Check sheet for the modelled part. Datum: model origin and axes. Units: mm. Face numbers are marked on the shaded views. A direction names the side the tool comes from. Give positions to 0.01 mm unless a question says otherwise; leave off trailing zeros. Write each loop counter-clockwise with the first axis right and the second up, starting at its lowest first coordinate (ties: lowest second). Pieces come first, ordered by that corner, then holes. Notation, with made-up numbers: (15.5, -13) -> (21.5, -13) arc R13 cw to (21.5, 5) -> close; hole circle Ø2 at (34.5, 1). An arc over 180 degrees is marked (long way). Use a Markdown table: item, result. Add a question column.
1. Cross-section at A-A (z = -0.85). Enter the section's corners in (x, y), then the cut area to 3 significant figures.
2. Scan lines: probe 1 along X at (y, z) = (39.5, 1); probe 2 along Y at (x, z) = (129.5, 1.25); probe 3 along X at (y, z) = (46, -0.25). Record each from-to range of solid material in increasing order. Write a range as [from, to].
3. Cross-section at D-D (y = 60.5). Enter the section's corners in (x, z).
4. Cross-section at B-B (x = 31.5). Enter the section's corners in (y, z).
5. Gauge pin test, flat ends, axial feed: P1, Ø1, axis at y = 38.5, z = -1, coming from the -X side; P2, Ø1.2, axis at y = 74, z = 0, coming from the +X side; P3, Ø3.5, axis at x = 3.5, y = 22, coming from the -Z side; P4, Ø1, axis at x = 32, y = 37, coming from the +Z side. Record the tip position at first contact, or that the pin passes through.
6. Set-up check for the marked faces 1 and 2: record each of +Z, -Z, +X, -X, +Y, -Y from which the full face is reachable in a straight line by a thin tool's end or side.
7. Cross-section at C-C (y = 39.5). Enter the section's corners in (x, z), then the cut area to 3 significant figures.
Autodesk Inventor part; units mm, degrees
ref_plane "YZ Plane" through (0, 0, 0) normal (1, 0, 0) x (0, 1, 0)
ref_plane "XZ Plane" through (0, 0, 0) normal (0, 1, 0) x (-1, 0, 0)
ref_plane "XY Plane" through (0, 0, 0) normal (0, 0, 1) x (1, 0, 0)
sketch "Sketch1" plane through (0, 0, 0) normal (0, 0, 1) x (1, 0, 0)
  line L0 (0, 0) -> (123, 0)
  line L1 (123, 0) -> (123, 79)
  line L2 (123, 79) -> (0, 79)
  line L3 (0, 79) -> (0, 0)
  line L4 (12, 79) -> (12, 0)
  line L5 (123, 69.5) -> (126.5, 69.5)
  line L6 (126.5, 69.5) -> (126.5, 9.5)
  line L7 (126.5, 9.5) -> (123, 9.5)
  line L8 (123, 9.5) -> (123, 69.5)
  line L9 (126.5, 9.5) -> (132.5, 9.5)
  line L10 (132.5, 9.5) -> (132.5, 69.5)
  line L11 (132.5, 69.5) -> (126.5, 69.5)
  line L12 (126.5, 69.5) -> (126.5, 9.5)
  line L13 (123, 69.5) -> (119, 69.5)
  line L14 (119, 69.5) -> (119, 79)
  line L15 (119, 79) -> (123, 79)
  line L16 (123, 79) -> (123, 69.5)
  line L17 (123, 9.5) -> (119, 9.5)
  line L18 (119, 9.5) -> (119, 0)
  line L19 (119, 0) -> (123, 0)
  line L20 (123, 0) -> (123, 9.5)
  circle A0 centre (129.5, 39.5) radius 2.1
  line L21 (9, 39.5) -> (5, 39.5) construction
  line L22 (9, 42) -> (5, 42)
  line L23 (5, 37) -> (9, 37)
  arc A1 (9, 37) -> (9, 42) centre (9, 39.5) ccw
  arc A2 (5, 42) -> (5, 37) centre (5, 39.5) ccw
  point P0 (7, 39.5)
  dimension "d0" = 123
  dimension "d1" = 79
  dimension "d2" = 111
  dimension "d3" = 3.5
  dimension "d4" = 6
  dimension "d5" = 60
  dimension "d6" = 9.5
  dimension "d7" = 4
  dimension "d8" = 4
  dimension "d9" = 4.2
  dimension "d10" = 3
  dimension "d11" = 30
  dimension "d20" = 5
  dimension "d21" = 3
  dimension "d22" = 4
  dimension "d23" = 39.5
extrude "Extrusion1" add sketch "Sketch1" along normal blind 2 contours L3 L2 L4 L0 | L4 L2 L14 L13 L1 L17 L18 L0 | L1 L5 L6 L7 | L6 L11 L10 L9 | A0
extrude "Extrusion3" add sketch "Sketch1" against normal blind 2 contours L4 L2 L14 L13 L1 L17 L18 L0 | L6 L11 L10 L9
sketch "Sketch2" plane through (0, 0, 2) normal (0, 0, 1) x (1, 0, 0)
  circle A0 centre (60, 39.5) radius 34
  line L0 (119, 79) -> (0, 79)
  line L1 (0, 79) -> (0, 0)
  line L2 (59, 52.5) -> (64, 52.5)
  line L3 (64, 52.5) -> (64, 47.5)
  line L4 (64, 47.5) -> (59, 47.5)
  line L5 (59, 47.5) -> (59, 52.5)
  line L6 (59, 31.5) -> (64, 31.5)
  line L7 (64, 31.5) -> (64, 26.5)
  line L8 (64, 26.5) -> (59, 26.5)
  line L9 (59, 26.5) -> (59, 31.5)
  circle A1 centre (33, 39.5) radius 1.5
  circle A2 centre (33, 39.5) radius 4
  line L10 (35, 42.9641) -> (35, 36.0359)
  line L11 (33, 41) -> (35, 41)
  line L12 (33, 38) -> (35, 38)
  circle A3 centre (33, 39.5) radius 5
  line L13 (35, 42.9641) -> (35, 44.0826)
  line L14 (35, 36.0359) -> (35, 34.9174)
  line L15 (35, 42.9641) -> (49, 42.9641)
  line L16 (49, 42.9641) -> (49, 36.0359)
  line L17 (49, 36.0359) -> (35, 36.0359)
  line L18 (35, 36.0359) -> (35, 42.9641)
  dimension "d24" = 68
  dimension "d25" = 39.5
  dimension "d26" = 60
  dimension "d27" = 16
  dimension "d28" = 5
  dimension "d29" = 5
  dimension "d30" = 8
  dimension "d31" = 5
  dimension "d32" = 31
  dimension "d33" = 27
  dimension "d34" = 3
  dimension "d35" = 8
  dimension "d36" = 64
  dimension "d37" = 2
  dimension "d38" = 10
  dimension "d51" = 16
  dimension "d52" = 6.9282
extrude "Extrusion4" [suppressed]
sketch "Sketch3" plane through (0, 0, 5.7) normal (0, 0, 1) x (1, 0, 0)
  line L0 (59, 52.5) -> (64, 52.5)
  line L1 (59, 52.5) -> (65.1, 52.5)
  line L2 (65.1, 52.5) -> (65.1, 47.5)
  line L3 (65.1, 47.5) -> (59, 47.5)
  line L4 (59, 47.5) -> (59, 52.5)
  line L5 (59, 47.5) -> (64, 47.5)
  line L6 (59, 31.5) -> (64, 31.5)
  line L7 (59, 31.5) -> (65.1, 31.5)
  line L8 (65.1, 31.5) -> (65.1, 26.5)
  line L9 (65.1, 26.5) -> (59, 26.5)
  line L10 (59, 26.5) -> (59, 31.5)
  line L11 (59, 26.5) -> (64, 26.5)
  line L12 (64, 47.5) -> (64, 52.5)
  line L13 (64, 26.5) -> (64, 31.5)
  point P0 (0, 0)
  point P1 (61.5, 47.5)
  point P2 (61.5, 26.5)
  dimension "d41" = 1.1
  dimension "d42" = 1.1
extrude "Extrusion5" [suppressed]
fillet "Fillet1" [suppressed]
extrude "Extrusion6" [suppressed]
sketch "Sketch4" plane through (0, 0, 6.5) normal (0, 0, 1) x (1, 0, 0)
  line L0 (35, 42.9641) -> (35, 36.0359)
  line L1 (33, 41) -> (35, 41)
  circle A0 centre (33, 39.5) radius 1.5
  line L2 (33, 38) -> (35, 38)
  arc A1 (35, 42.9641) -> (35, 36.0359) centre (33, 39.5) ccw
  point P0 (0, 0)
extrude "Extrusion7" [suppressed]
fillet "Fillet2" [suppressed]
extrude "Extrusion8" [suppressed]
fillet "Fillet3" [suppressed]
sketch "Sketch5" plane through (0, 0, 2) normal (0, 0, 1) x (1, 0, 0)
  point P0 (0, 0)
extrude "Extrusion9" cut sketch "Sketch1" along normal through all both and the other way through all contours A0
sketch "Sketch6" plane through (0, 0, 2) normal (0, 0, 1) x (1, 0, 0)
  line L0 (7, 39.5) -> (129.5, 39.5) construction
  line L1 (20, 39.5) -> (40, 39.5) construction
  line L2 (20, 35.5) -> (40, 35.5)
  line L3 (40, 43.5) -> (20, 43.5)
  arc A0 (20, 43.5) -> (20, 35.5) centre (20, 39.5) ccw
  arc A1 (40, 35.5) -> (40, 43.5) centre (40, 39.5) ccw
  line L4 (0, 79) -> (0, 0)
  point P0 (30, 39.5)
  dimension "d58" = 8
  dimension "d59" = 20
  dimension "d60" = 20
extrude "Extrusion10" cut sketch "Sketch6" against normal through all
equation "\"d6\" = -0.5 * d5 + 0.5 * d1"
equation "\"d10\" = 0.5 * d4"
equation "\"d11\" = 0.5 * d5"
equation "\"d25\" = d23"
equation "\"d29\" = d28"
equation "\"d30\" = 0.5 * d27"
properties part number "gps_cover_flat_only"
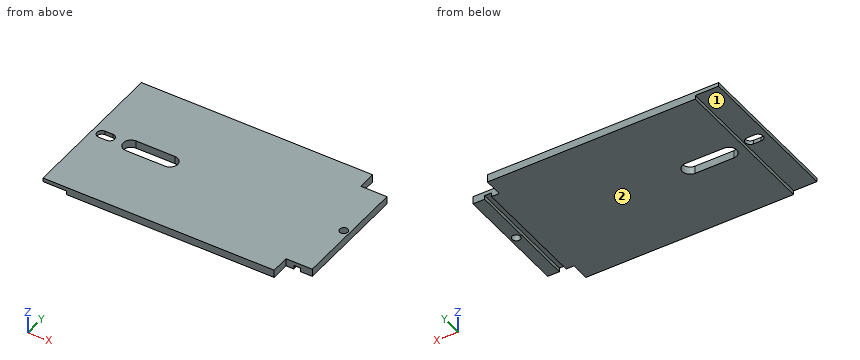
Worked answers:
| question | item | result |
|---|---|---|
| 1 | outline | (12, 0) -> (119, 0) -> (119, 9.5) -> (123, 9.5) -> (123, 69.5) -> (119, 69.5) -> (119, 79) -> (12, 79) -> close; (126.5, 9.5) -> (132.5, 9.5) -> (132.5, 69.5) -> (126.5, 69.5) -> close; hole (20, 35.5) -> (40, 35.5) arc R4 ccw to (40, 43.5) -> (20, 43.5) arc R4 ccw to start; hole circle Ø4.2 at (129.5, 39.5) |
| 1 | area | 8,830 mm² |
| 2 | probe 1 | x = [0, 2.5], [11.5, 16], [44, 127.4], [131.6, 132.5] |
| 2 | probe 2 | y = [9.5, 37.4], [41.6, 69.5] |
| 2 | probe 3 | x = [12, 123], [126.5, 132.5] |
| 3 | outline | (0, 0) -> (12, 0) -> (12, -2) -> (123, -2) -> (123, 0) -> (126.5, 0) -> (126.5, -2) -> (132.5, -2) -> (132.5, 2) -> (0, 2) -> close |
| 4 | outline | (0, -2) -> (35.5, -2) -> (35.5, 2) -> (0, 2) -> close; (43.5, -2) -> (79, -2) -> (79, 2) -> (43.5, 2) -> close |
| 5 | P1 | stops at x = 12 |
| 5 | P2 | stops at x = 119 |
| 5 | P3 | stops at z = 0 |
| 5 | P4 | passes through |
| 6 | face 1 | -Z, -X, +Y, -Y |
| 6 | face 2 | -Z, +X, -X, +Y, -Y |
| 7 | outline | (0, 0) -> (2.5, 0) -> (2.5, 2) -> (0, 2) -> close; (11.5, 0) -> (12, 0) -> (12, -2) -> (16, -2) -> (16, 2) -> (11.5, 2) -> close; (44, -2) -> (123, -2) -> (123, 0) -> (126.5, 0) -> (126.5, -2) -> (127.4, -2) -> (127.4, 2) -> (44, 2) -> close; (131.6, -2) -> (132.5, -2) -> (132.5, 2) -> (131.6, 2) -> close |
| 7 | area | 352 mm² |
